Design review of the part shown in the three views and the two pictorial views. Dimensions are in mm from the part's minimum x, y and z. A direction names the side the tool comes from. Coordinates: 2 decimals unless noted, no trailing zeros. Order: outer loops, then holes, each group sorted by start corner. A loop starts at its lowest first (then second) coordinate and runs counter-clockwise, first axis right, second up. Notation, with made-up numbers: M -9.75,64 L -2.75,64 A22 cw -2.75,93 Z; hole C 16,-2.75 d4. An arc over 180 degrees is marked long. Use CSV: the item, a comma, the result in double quotes.
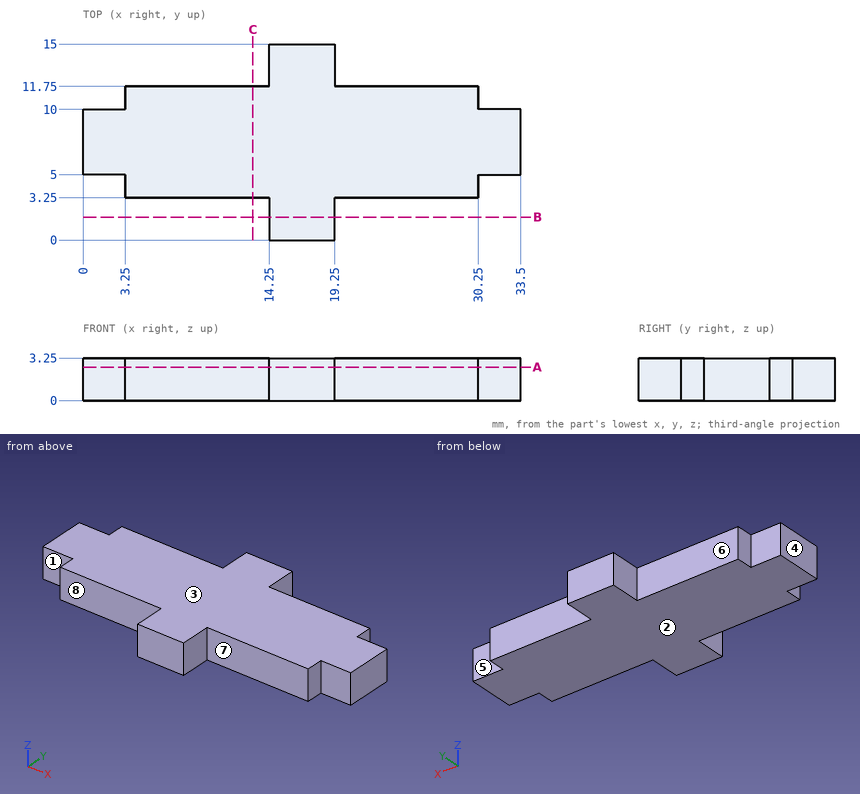
(1) Add section C-C on x = 13. State the section outline as (y, z) points.
The answers:
outline,"M 3.25,0 L 11.75,0 L 11.75,3.25 L 3.25,3.25 Z"
(2) Add section A-A on z = 2.55. State the section outline as (x, y) points, and give its area (4 significant figures).
The answers:
outline,"M 0,5 L 3.25,5 L 3.25,3.25 L 14.25,3.25 L 14.25,0 L 19.25,0 L 19.25,3.25 L 30.25,3.25 L 30.25,5 L 33.5,5 L 33.5,10 L 30.25,10 L 30.25,11.75 L 19.25,11.75 L 19.25,15 L 14.25,15 L 14.25,11.75 L 3.25,11.75 L 3.25,10 L 0,10 Z"
area,"294.5 mm2"
(3) Wall thickness on probe 1 along Y at (x, z) = (23, 0.9); probe 2 along X at (y, z) = (13, 2.4); probe 3 along X at (y, z) = (10.75, 2.9): over which ranges is each line inside the solid? List them lowest first.
The answers:
probe 1,"y = 3.25 to 11.75"
probe 2,"x = 14.25 to 19.25"
probe 3,"x = 3.25 to 30.25"
(4) Clearance check with flat-ended pins moving along their axes: P1, Ø1.6, axis at x = 26.5, z = 2, coming from the -Y side; P2, Ø8, axis at x = 9.5, y = 9.5, coming from the -Z side; P3, Ø0.9, axis at y = 4, z = 2, coming from the +X side; P4, Ø1, axis at y = 1.5, z = 1.5, coming from the -X side. State where each tip first meets the part, or that it passes through.
The answers:
P1,"stops at y = 3.25"
P2,"stops at z = 0"
P3,"stops at x = 30.25"
P4,"stops at x = 14.25"
(5) The part is to be moulded in two halves that separate along Z. For the marked faces 1, 2 and 3, say which applies: pulls with the +Z half, pulls with the -Z half, needs draft (parallel to the pull), parting line crosses it, or undercut.
The answers:
face 1,"needs draft"
face 2,"pulls with the -Z half"
face 3,"pulls with the +Z half"
(6) For the marked faces 4, 5, 6, 7 and 8, list the 3-axis set-ups (+Z, -Z, +X, -X, +Y, -Y) from which the entire face can be reached by the end or side of a thin tool; tool diameter is ignored.
The answers:
face 4,"+Z, -Z, -X, +Y, -Y"
face 5,"+Z, -Z, +X, +Y"
face 6,"+Z, -Z, -X, +Y"
face 7,"+Z, -Z, +X, -Y"
face 8,"+Z, -Z, -X, -Y"
(7) Add section B-B on y = 1.75. State the section outline as (x, z) points.
The answers:
outline,"M 14.25,0 L 19.25,0 L 19.25,3.25 L 14.25,3.25 Z"
